Input: part model. Units: mm. Frame: model coordinates. A direction names the side the tool comes from. Coordinates: 2 decimals unless noted, no trailing zeros. Write each loop counter-clockwise with the first axis right and the second up, starting at its lowest first coordinate (ties: lowest second). Pieces come first, ordered by that corner, then holes. Notation, with made-up numbers: M 41.25,-32 L 67.25,-32 A28 cw 67.25,-3 Z; hole C -35.5,-0.75 d2. An arc over 180 degrees is marked long. Write each question's results on one line, items separated by ' | '. Start each with the question number.
1. Section query A-A, the plane x = 19. Output: boundary loops of the cut face in (y, z).
2. First-contact query: pin 1 (0.8 mm diameter, centred on x = 7, y = 1.5, fed in from -Z); pin 2 (3.5 mm diameter, centred on x = 34.8, z = 22.3, fed in from +Y). Flat tips, straight axial feed; report the tip coordinate or a pass-through.
3. Ray query, probe 1 along X at (y, z) = (0.8, 22.3); probe 2 along Z at (x, y) = (-28.5, 1.45); probe 3 along X at (y, z) = (1.35, -2.5). Return the intervals inside material, ascending.
4. Pull-direction query (X, two-part tool) for faces 1 (the flat face through (-33.1, 1.5, 20.6)), 2 (the flat face through (33.1, 1.5, -20.6)), 3 (the cylindrical face through (34.379, 0.507, 23.316)); classes: +X half, -X half, draft (parallel to the pull), parting line (faces both ways), or undercut.
5. Section query B-B, the plane y = 1.4. Output: boundary loops of the cut face in (x, z), and give its area (3 significant figures).
6. Set-up query: faces 4 (the flat face through (-3, 1, 23)), 5 (the flat face through (-33.1, 1.5, -20.6)), 6 (the flat face through (33.1, 1.5, 20.6)). Return all of +Z, -Z, +X, -X, +Y, -Y with unobstructed straight access to the full face (end or side cutting, diameter ignored); none if empty.
```python
from build123d import *

# Parameters (mm, degrees)
SKETCH1_W           = 74
SKETCH1_H           = 49
BOSS_EXTRUDE1_DEPTH = 1
SKETCH2_W           = 69.5
SKETCH2_H           = 44.5
BOSS_EXTRUDE2_DEPTH = 1
CHAMFER1_SIZE       = 2
CHAMFER2_SIZE       = 3.3
SKETCH3_R           = 1.1
CUT_EXTRUDE1_DEPTH  = 1


with BuildPart() as part:
    # Sketch1 → Boss-Extrude1 (new body)
    with BuildSketch(Plane(origin=(0, 0, 0), x_dir=(1, 0, 0), z_dir=(0, 1, 0))):
        Rectangle(SKETCH1_W, SKETCH1_H)
    extrude(amount=BOSS_EXTRUDE1_DEPTH)

    # Sketch2 → Boss-Extrude2 (add)
    with BuildSketch(Plane(origin=(0, 1, 0), x_dir=(1, 0, 0), z_dir=(0, 1, 0))):
        Rectangle(SKETCH2_W, SKETCH2_H)
    extrude(amount=BOSS_EXTRUDE2_DEPTH)

    # Chamfer1
    chamfer1_edges = [part.edges().sort_by_distance(p)[0] for p in [
        (37, 0.5, 24.5),
        (-37, 0.5, 24.5),
        (-37, 0.5, -24.5),
        (37, 0.5, -24.5),
    ]]
    chamfer(chamfer1_edges, length=CHAMFER1_SIZE)

    # Chamfer2
    chamfer2_edges = [part.edges().sort_by_distance(p)[0] for p in [
        (34.75, 1.5, 22.25),
        (34.75, 1.5, -22.25),
        (-34.75, 1.5, -22.25),
        (-34.75, 1.5, 22.25),
    ]]
    chamfer(chamfer2_edges, length=CHAMFER2_SIZE)

    # Sketch3 → Cut-Extrude1 (cut)
    with BuildSketch(Plane(origin=(0, 1, 0), x_dir=(1, 0, 0), z_dir=(0, 1, 0))):
        with Locations(Location((-34.8, 22.3, 0), (0, 0, 270))):
            Circle(SKETCH3_R)
        with Locations(Location((34.8, 22.3, 0), (0, 0, 270))):
            Circle(SKETCH3_R)
        with Locations(Location((34.8, -22.3, 0), (0, 0, 270))):
            Circle(SKETCH3_R)
        with Locations(Location((-34.8, -22.3, 0), (0, 0, 270))):
            Circle(SKETCH3_R)
    extrude(amount=-CUT_EXTRUDE1_DEPTH, mode=Mode.SUBTRACT)


solid = part.part
```
Answer:
1) outline: M 0,-24.5 L 1,-24.5 L 1,-22.25 L 2,-22.25 L 2,22.25 L 1,22.25 L 1,24.5 L 0,24.5 Z
2) pin 1: z = -22.25 | pin 2: y = 1
3) probe 1: -37 to -35.9, -33.7 to 33.7, 35.9 to 37 | probe 2: -22.25 to 22.25 | probe 3: -34.75 to 34.75
4) face 1: -X half | face 2: +X half | face 3: undercut
5) outline: M -34.75,-18.95 L -31.45,-22.25 L 31.45,-22.25 L 34.75,-18.95 L 34.75,18.95 L 31.45,22.25 L -31.45,22.25 L -34.75,18.95 Z | area: 3,070 mm^2
6) face 4: +Y | face 5: -Z, -X, +Y | face 6: +Z, +X, +Y
